Read the model definition and answer for the solid it produces. Units are mm, in the model's axes. Face numbers are marked on the shaded views. A direction names the side the tool comes from. Coordinates: 2 decimals unless noted, no trailing zeros. Order: outer loops, then holes, each group sorted by start corner. A loop starts at its lowest first (then second) coordinate and runs counter-clockwise, first axis right, second up.
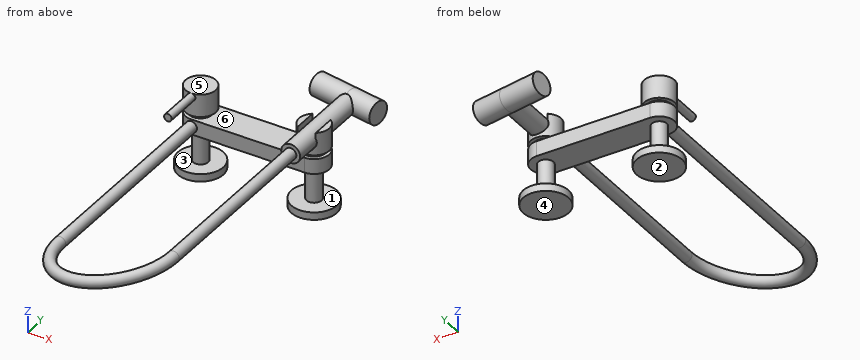
from build123d import *

# Parameters (mm, degrees)
SKETCH_1_R               = 30
EXTRUDE_1_DEPTH          = 10
EXTRUDE_1_2_DEPTH        = 10
SKETCH_2_R               = 10
EXTRUDE_2_DEPTH          = 45
EXTRUDE_3_DEPTH          = 20
SKETCH_4_R               = 15
EXTRUDE_4_DEPTH          = 5
SKETCH_5_R               = 20
EXTRUDE_5_DEPTH          = 30
SKETCH_6_R               = 5
EXTRUDE_6_DEPTH          = 70
CUT_EXTRUDE_1_DEPTH      = 223.26110779
CUT_EXTRUDE_1_DEPTH_BACK = 223.26110779
SKETCH_9_R               = 7.5
EXTRUDE_7_DEPTH          = 50
SWEEP_START              = -300.0000001
SWEEP_1_OUTLINE_R        = 7.5
SWEEP_1_DEPTH            = 300.0000001
SWEEP_1_2_OUTLINE_R      = 7.5
SWEEP_1_2_ANGLE          = 180
EXTRUDE_8_DEPTH          = 80
EXTRUDE_8_DEPTH_BACK     = 50
SKETCH_10_R              = 12.5
SWEEP_2_PROFILE_R        = 15


with BuildPart() as part:
    # Sketch 1 → Extrude 1 (new body)
    with BuildSketch(Plane.XY):
        Circle(SKETCH_1_R)
    extrude(amount=EXTRUDE_1_DEPTH)



with BuildPart() as body_2:
    # Sketch 1 → Extrude 1 2 (new body)
    with BuildSketch(Plane.XY):
        with Locations((150, 0)):
            Circle(SKETCH_1_R)
    extrude(amount=EXTRUDE_1_2_DEPTH)


with BuildPart() as part_1:
    add(part.part)

    add(body_2.part)  # Extrude 2 merges body 2
    # Sketch 2 → Extrude 2 (add)
    with BuildSketch(Plane.XY.offset(10)):
        with Locations(Location((0, 0, 0), (0, 0, 180))):
            Circle(SKETCH_2_R)
        with Locations(Location((150, 0, 0), (0, 0, 180))):
            Circle(SKETCH_2_R)
    extrude(amount=EXTRUDE_2_DEPTH)

    # Sketch 3 → Extrude 3 (add)
    with BuildSketch(Plane.XY.offset(55)):
        with BuildLine():
            Line((0, 20), (150, 20))
            ThreePointArc((150, 20), (170, 0), (150, -20))
            Line((150, -20), (0, -20))
            ThreePointArc((0, -20), (-20, 0), (0, 20))
        make_face()
    extrude(amount=EXTRUDE_3_DEPTH)

    # Sketch 4 → Extrude 4 (add)
    with BuildSketch(Plane.XY.offset(75)):
        Circle(SKETCH_4_R)
        with Locations((150, 0)):
            Circle(SKETCH_4_R)
    extrude(amount=EXTRUDE_4_DEPTH)

    # Sketch 5 → Extrude 5 (add)
    with BuildSketch(Plane.XY.offset(80)):
        Circle(SKETCH_5_R)
        with Locations((150, 0)):
            Circle(SKETCH_5_R)
    extrude(amount=EXTRUDE_5_DEPTH)

    # Sketch 6 → Extrude 6 (add)
    with BuildSketch(Plane(origin=(0, 0, 0), x_dir=(1, 0, 0), z_dir=(0, 1, 0))):
        with Locations(Location((0, -105, 0), (0, 0, 270))):
            Circle(SKETCH_6_R)
    extrude(amount=-EXTRUDE_6_DEPTH)

    # Sketch 8 → Cut-Extrude 1 (cut, two sides: drawn at the far end of the back side and taken through both)
    with BuildSketch(Plane(origin=(0, 0, 0), x_dir=(1, 0, 0), z_dir=(0, 1, 0)).offset(-CUT_EXTRUDE_1_DEPTH_BACK)):
        with BuildLine():
            Line((138, -102), (138, -110))
            Line((138, -110), (162, -110))
            Line((162, -110), (162, -102))
            ThreePointArc((162, -102), (150, -84), (138, -102))
        make_face()
    extrude(amount=CUT_EXTRUDE_1_DEPTH + CUT_EXTRUDE_1_DEPTH_BACK, mode=Mode.SUBTRACT)

    # Sketch 9 → Extrude 7 (add)
    with BuildSketch(Plane(origin=(0, 0, 0), x_dir=(1, 0, 0), z_dir=(0, 1, 0))):
        with Locations(Location((0, -65, 0), (0, 0, 270))):
            Circle(SKETCH_9_R)
    extrude(amount=-EXTRUDE_7_DEPTH)

    # Sweep 1: read off the stored shape, not the designer's step
    # Sweep 1 outline → Sweep 1 (add)
    with BuildSketch(Plane(origin=(0, 0, 0), x_dir=(1, 0, 0), z_dir=(0, 1, 0)).offset(SWEEP_START)):
        with Locations((0, -65)):
            Circle(SWEEP_1_OUTLINE_R)
        with Locations((150, -97)):
            Circle(SWEEP_1_OUTLINE_R)
    extrude(amount=SWEEP_1_DEPTH)

    # Sweep 1 2 outline → Sweep 1 2 (revolve)
    with BuildSketch(Plane(origin=(88.263050502, -300, 18.829450774), x_dir=(0.9779928364243075, 0, 0.20863847177051914), z_dir=(0, 1, 0))):
        with Locations((76.68767828, -63.569534368)):
            Circle(SWEEP_1_2_OUTLINE_R)
    revolve(axis=Axis((88.263050502, -300, 18.829450774), (0.20863847177051914, 0, -0.9779928364243075)), revolution_arc=SWEEP_1_2_ANGLE)

    # Sketch 10 → Extrude 8 (add, two sides: drawn at the far end of the back side and taken through both)
    with BuildSketch(Plane(origin=(0, 0, 0), x_dir=(1, 0, 0), z_dir=(0, 1, 0)).offset(-EXTRUDE_8_DEPTH_BACK)):
        with Locations(Location((150, -97, 0), (0, 0, 270))):
            Circle(SKETCH_10_R)
    extrude(amount=EXTRUDE_8_DEPTH + EXTRUDE_8_DEPTH_BACK)

    # Sweep 2: sweep along a path in Sketch 11
    with BuildLine(Plane.XY.offset(97)) as sweep_2_path:
        Line((189.39231012, 73.054072893), (150, 80))
        Line((150, 80), (100.759612349, 88.682408883))
    # Sweep 2 profile (on start of the path) → Sweep 2 (sweep)
    with BuildSketch(Plane(origin=(189.39231012, 73.054072893, 97), x_dir=(-0.17364817766693041, -0.9848077530122081, 0), z_dir=(-0.9848077530122081, 0.17364817766693041, 0))):
        Circle(SWEEP_2_PROFILE_R)
    sweep(path=sweep_2_path.line)


solid = part_1.part
Q1. Each of these flat-tipped pins is pushed along its axis until it touches: P1, Ø5, axis at x = -2.5, z = 104.5, coming from the -Y side; P2, Ø23.5, axis at x = 150, z = 97, coming from the +Y side; P3, Ø5, axis at y = -314.5, z = 74, coming from the +X side. Where does it stop, or does it pass through?
Q2. Straight lines are drawn through the part: L1, parallel to Z at x = 150, y = -11; L2, parallel to X at y = -2, z = 97; L3, parallel to Z at x = 150, y = -1.5. For each, find the intervals that lie inside material, in ascending order.
Q3. The part is cut by section B-B, the plane z = 46. Determine the outline of the cut face in (x, y), then the cut area to 3 significant figures.
Q4. Which of the six approach directions +Z, -Z, +X, -X, +Y, -Y give full straight-line access (tool end or side, diameter ignored) to the marked faces 1 and 2?
Q5. The part is cut by section C-C, the plane y = 53. Determine the outline of the cut face in (x, z), then the cut area to 3 significant figures.
Q6. The part is cut by section A-A, the plane y = -169. Determine the outline of the cut face in (x, z), then the cut area to 3 significant figures.
Q7. Determine the mould class of the marked faces 3, 4, 5 and 6 for opening direction Z: +Z half, -Z half, draft (parallel to the pull), parting line (faces both ways), or undercut.
Computed values:
1. P1: stops at y = -70
1. P2: stops at y = 97.3
1. P3: stops at x = 5.76
2. L1: z = 0 to 10, 55 to 84, 84.5 to 109.5
2. L2: x = -19.9 to 19.9, 130.1 to 137, 137.5 to 162.5, 163 to 169.9
2. L3: z = 0 to 84, 84.5 to 109.5
3. outline: circle Ø20 at (0, 0); circle Ø20 at (150, 0)
3. area: 628 mm2
4. face 1: none
4. face 2: -Z, +X, -X, +Y, -Y
5. outline: circle Ø25 at (150, 97)
5. area: 491 mm2
6. outline: circle Ø15 at (0, 65); circle Ø15 at (150, 97)
6. area: 353 mm2
7. face 3: undercut
7. face 4: -Z half
7. face 5: +Z half
7. face 6: undercut
